Part model, mm, in its own coordinate system. Round coordinates to 2 decimals unless told otherwise and drop trailing zeros. Write each loop counter-clockwise with the first axis right and the second up, starting at its lowest first coordinate (ties: lowest second). Pieces come first, ordered by that corner, then holes. Notation, with made-up numbers: M 46,2 L 90,2 A21 ccw 90,8 Z; hole C 78,-28.75 d9. An arc over 180 degrees is marked long. Use one line per item in the form item = value. Start each with the question number.
Item 1: Cut at A-A, the plane x = 0. Give the cut face in (y, z) (3 decimals).
Item 2: Probe L1, parallel to Y at x = 0, z = 0.6 (3 decimals); L2, parallel to Y at x = 41, z = 1.2; L3, parallel to Y at x = -34, z = 0.4. List the from-to ranges inside material, lowest first.
Item 3: Flat gauge pins, fed straight in: pin 1 Ø1 at (y, z) = (-14, 0.5) entering from -X; pin 2 Ø1 at (y, z) = (-55.5, 1) entering from -X; pin 3 Ø1.5 at (x, z) = (9, 1.5) entering from -Y. Where does each tip first touch, or does it go through?
from build123d import *

# Parameters (mm, degrees)
SKETCH1_R           = 85.725
BOSS_EXTRUDE2_DEPTH = 2.54


with BuildPart() as part:
    # Sketch1 → Boss-Extrude2 (new body)
    with BuildSketch(Plane.XY):
        Circle(SKETCH1_R)
        with BuildLine():
            ThreePointArc((-50.476604824, -65.319329952), (2.284509609, 82.518382896), (46.785345693, -68.012013118))
            ThreePointArc((46.785345693, -68.012013118), (46.595439838, -67.75364435), (46.380442263, -67.515747951))
            Line((46.380442263, -67.515747951), (29.451630282, -50.58693597))
            ThreePointArc((29.451630282, -50.58693597), (24.961502222, -50.58693597), (24.961502222, -55.07706403))
            Line((24.961502222, -55.07706403), (41.33826935, -71.453831158))
            ThreePointArc((41.33826935, -71.453831158), (-2.304078902, -82.517838801), (-45.26104742, -69.035788447))
            Line((-45.26104742, -69.035788447), (-31.302323003, -55.07706403))
            ThreePointArc((-31.302323003, -55.07706403), (-31.302323003, -50.58693597), (-35.792451064, -50.58693597))
            Line((-35.792451064, -50.58693597), (-50.172516759, -64.967001665))
            ThreePointArc((-50.172516759, -64.967001665), (-50.331025251, -65.137586452), (-50.476604824, -65.319329952))
        make_face(mode=Mode.SUBTRACT)
    extrude(amount=BOSS_EXTRUDE2_DEPTH)


solid = part.part
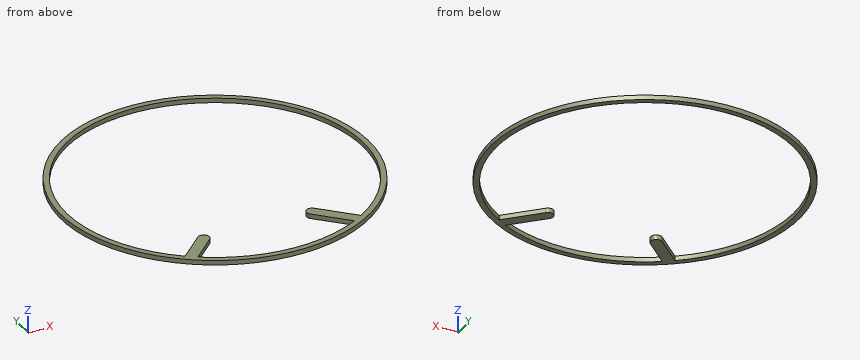
Model answer:
q1.outline = M -85.725,0 L -82.55,0 L -82.55,2.54 L -85.725,2.54 Z; M 82.55,0 L 85.725,0 L 85.725,2.54 L 82.55,2.54 Z
q2.L1 = -85.725 to -82.55, 82.55 to 85.725
q2.L2 = -75.28 to -71.65, -71.12 to -62.14, 71.65 to 75.28
q2.L3 = -78.69 to -75.22, -57.77 to -49.69, 75.22 to 78.69
q3.pin_1 = -84.66
q3.pin_2 = -65.76
q3.pin_3 = -85.33
